The listing builds one solid part. Answer for the finished solid, in the listing's coordinates (mm). Round coordinates to 2 decimals unless told otherwise and drop trailing zeros. Order: outer loops, then holes, each group sorted by start corner. A loop starts at its lowest first (then second) coordinate and runs counter-clockwise, first axis right, second up. Notation, with made-up numbers: (-10, 23.5) -> (24, 23.5) arc R12 cw to (24, 28.5) -> close; hole circle Ø9 at (-23.75, 80.5). An arc over 180 degrees is marked (long way). Answer in a Markdown table with one row per item. Add a question column.
```python
from build123d import *

# Parameters (mm, degrees)
CROQUIS1_R              = 2.75
SALIENTE_EXTRUIR1_DEPTH = 1
CROQUIS2_R              = 2.45
SALIENTE_EXTRUIR2_DEPTH = 5.05
C_PULA1_FACE_RADIUS     = 2.45
C_PULA1_HEIGHT          = 2.45
CROQUIS3_R              = 0.25
SALIENTE_EXTRUIR3_DEPTH = 25.5
CROQUIS5_R              = 0.25
SALIENTE_EXTRUIR5_DEPTH = 27


with BuildPart() as part:
    # Croquis1 → Saliente-Extruir1 (new body)
    with BuildSketch(Plane(origin=(0, 0, 0), x_dir=(1, 0, 0), z_dir=(0, 1, 0))):
        Circle(CROQUIS1_R)
    extrude(amount=SALIENTE_EXTRUIR1_DEPTH)

    # Croquis2 → Saliente-Extruir2 (add)
    with BuildSketch(Plane(origin=(0, 1, 0), x_dir=(1, 0, 0), z_dir=(0, 1, 0))):
        Circle(CROQUIS2_R)
    extrude(amount=SALIENTE_EXTRUIR2_DEPTH)

    # C_pula1: a dome of height H over a round flat face of radius A is a cap of a sphere of radius (A * A + H * H) / (2 * H)
    c_pula1_r = (C_PULA1_FACE_RADIUS * C_PULA1_FACE_RADIUS + C_PULA1_HEIGHT * C_PULA1_HEIGHT) / (2 * C_PULA1_HEIGHT)
    c_pula1_base = Plane((0, 6.05, 0), z_dir=(0, 1, 0))
    with Locations(c_pula1_base.offset(C_PULA1_HEIGHT - c_pula1_r)):
        c_pula1_ball = Sphere(c_pula1_r, mode=Mode.PRIVATE)
    add(split(c_pula1_ball, bisect_by=c_pula1_base, keep=Keep.TOP, mode=Mode.PRIVATE))

    # Croquis3 → Saliente-Extruir3 (add)
    with BuildSketch(Plane.XZ):
        with Locations((-1.205162028, 0)):
            Circle(CROQUIS3_R)
    extrude(amount=SALIENTE_EXTRUIR3_DEPTH)

    # Croquis5 → Saliente-Extruir5 (add)
    with BuildSketch(Plane.XZ):
        with Locations((1.205162028, 0)):
            Circle(CROQUIS5_R)
    extrude(amount=SALIENTE_EXTRUIR5_DEPTH)


solid = part.part
```
Item 1: For a pull along Y with two mould halves and no side action, classify faces 1 (the face through (0, 0, 0)), 2 (the face through (-0.596, 0.493, 2.685)) as released by +Y, released by -Y, zero draft, split by the parting line, or undercut.
Item 2: The part is cut by section B-B, the plane y = -7. Give the vertices of the cut face in (x, z).
Item 3: Flat-ended cylindrical pins translate along their axes: P1, Ø3, axis at y = 3, z = 1.5, coming from the -X side; P2, Ø2, axis at y = -15, z = 0, coming from the -X side; P3, Ø1, axis at x = 2, y = -23, coming from the +Z side; P4, Ø1, axis at x = -1.5, z = 0.5, coming from the -Y side. Find the tip coordinate at first contact, or state that the pin passes through.
Item 4: The part is cut by section C-C, the plane z = 1.85. Give the vertices of the cut face in (x, y).
Item 5: Find the intervals of material crossed by probe 1 along Y at (x, z) = (1.9, -1.6); probe 2 along X at (y, z) = (-4.5, 0.15); probe 3 along Y at (x, z) = (-0.85, 2), in increasing order. Write a range as [from, to].
Item 6: The part is cut by section A-A, the plane x = 0. Give the vertices of the cut face in (y, z).
Resolved:
| question | item | result |
|---|---|---|
| 1 | face 1 | released by -Y |
| 1 | face 2 | zero draft |
| 2 | outline | circle Ø0.5 at (-1.21, 0); circle Ø0.5 at (1.21, 0) |
| 3 | P1 | x = -2.45 |
| 3 | P2 | x = -1.46 |
| 3 | P3 | through |
| 3 | P4 | y = -25.5 |
| 4 | outline | (-2.03, 0) -> (2.03, 0) -> (2.03, 1) -> (1.61, 1) -> (1.61, 6.05) arc R1.61 ccw to (-1.61, 6.05) -> (-1.61, 1) -> (-2.03, 1) -> close |
| 5 | probe 1 | [0, 1] |
| 5 | probe 2 | [-1.41, -1.01], [1.01, 1.41] |
| 5 | probe 3 | [0, 7.18] |
| 6 | outline | (0, -2.75) -> (1, -2.75) -> (1, -2.45) -> (6.05, -2.45) arc R2.45 ccw to (6.05, 2.45) -> (1, 2.45) -> (1, 2.75) -> (0, 2.75) -> close |
